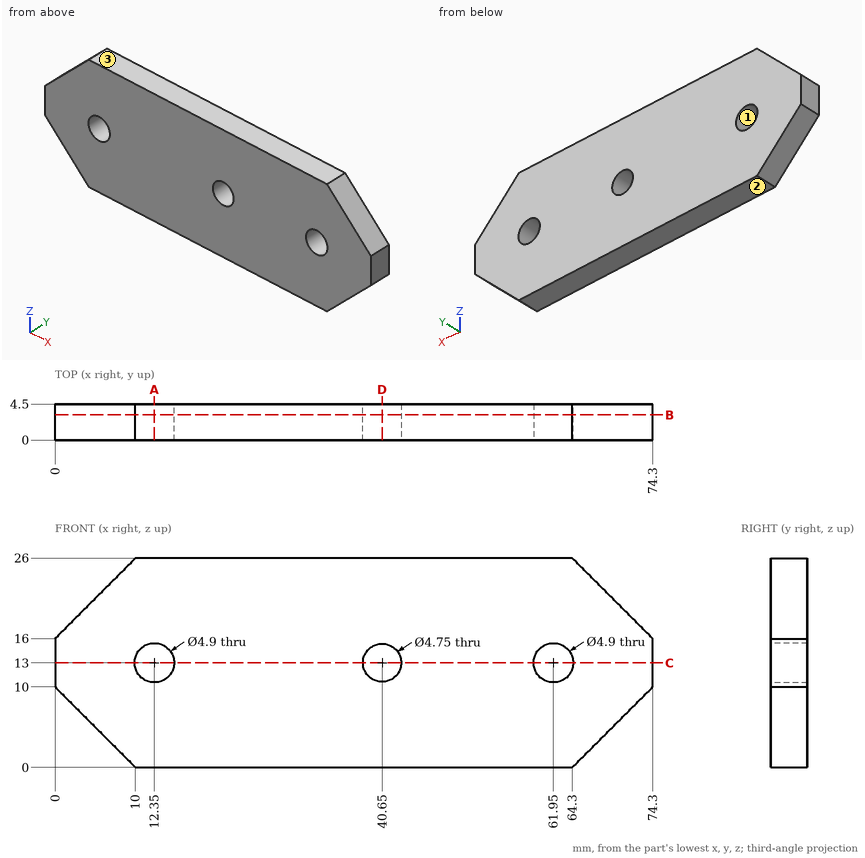
For this review, use the dimensioned drawing (mm, ordinates from the lowest corner) and the shaded views. Coordinates: 2 decimals unless noted, no trailing zeros. Loops run counter-clockwise (first coordinate to the right, second up) from the corner with the lowest first, then second, coordinate; pieces in that order, holes last. Notation, with made-up numbers: (-30, 67) -> (-20, 67) arc R19 cw to (-20, 89) -> close; hole circle Ø9 at (79.25, -33.5). An arc over 180 degrees is marked (long way). Use a Markdown table: item, result. Add a question column.
1. Draft analysis for pull direction Z (two halves, no side actions). For the marked faces 1, 2 and 3, state which applies: pulls with the +Z half, pulls with the -Z half, needs draft (parallel to the pull), parting line crosses it, or undercut.
2. To check wall thickness, follow line 1 (X direction, y = 2.9, z = 13) (3 decimals); line 2 (Z direction, x = 40.65, y = 3) (3 decimals); line 3 (X direction, y = 1.25, z = 12.25). State the ranges of each line that lie inside material, in increasing order.
3. Add section C-C on z = 13. Write out the cut boundary in (x, y) (3 decimals), plus the area to 3 significant figures.
4. Add section D-D on x = 40.65. Write out the cut boundary in (y, z) (3 decimals), plus the area to 3 significant figures.
5. Clearance check with a flat-ended pin moving along its axis: pin 1 Ø2 at (y, z) = (4, 19.5) entering from +X. State where the tip first meets the part, or that it passes through.
6. Add section B-B on y = 3.15. Write out the cut boundary in (x, z) (3 decimals), plus the area to 3 significant figures.
7. Add section A-A on x = 12.35. Write out the cut boundary in (y, z).
Returned:
| question | item | result |
|---|---|---|
| 1 | face 1 | undercut |
| 1 | face 2 | pulls with the -Z half |
| 1 | face 3 | pulls with the +Z half |
| 2 | line 1 | x = 0 to 9.9, 14.8 to 38.275, 43.025 to 59.5, 64.4 to 74.3 |
| 2 | line 2 | z = 0 to 10.625, 15.375 to 26 |
| 2 | line 3 | x = 0 to 10.02, 14.68 to 38.4, 42.9 to 59.62, 64.28 to 74.3 |
| 3 | outline | (0, 0) -> (9.9, 0) -> (9.9, 4.5) -> (0, 4.5) -> close; (14.8, 0) -> (38.275, 0) -> (38.275, 4.5) -> (14.8, 4.5) -> close; (43.025, 0) -> (59.5, 0) -> (59.5, 4.5) -> (43.025, 4.5) -> close; (64.4, 0) -> (74.3, 0) -> (74.3, 4.5) -> (64.4, 4.5) -> close |
| 3 | area | 269 mm² |
| 4 | outline | (0, 0) -> (4.5, 0) -> (4.5, 10.625) -> (0, 10.625) -> close; (0, 15.375) -> (4.5, 15.375) -> (4.5, 26) -> (0, 26) -> close |
| 4 | area | 95.6 mm² |
| 5 | pin 1 | stops at x = 71.8 |
| 6 | outline | (0, 10) -> (10, 0) -> (64.3, 0) -> (74.3, 10) -> (74.3, 16) -> (64.3, 26) -> (10, 26) -> (0, 16) -> close; hole circle Ø4.9 at (12.35, 13); hole circle Ø4.75 at (40.65, 13); hole circle Ø4.9 at (61.95, 13) |
| 6 | area | 1,680 mm² |
| 7 | outline | (0, 0) -> (4.5, 0) -> (4.5, 10.55) -> (0, 10.55) -> close; (0, 15.45) -> (4.5, 15.45) -> (4.5, 26) -> (0, 26) -> close |
